Autodesk Inventor part; units mm, degrees
ref_plane "YZ Plane" through (0, 0, 0) normal (1, 0, 0) x (0, 1, 0)
ref_plane "XZ Plane" through (0, 0, 0) normal (0, 1, 0) x (-1, 0, 0)
ref_plane "XY Plane" through (0, 0, 0) normal (0, 0, 1) x (1, 0, 0)
sketch "Náčrt1" plane through (0, 0, 0) normal (0, 1, 0) x (-1, 0, 0)
  line L0 (0, 0) -> (-75, 0)
  line L1 (-75, 0) -> (-75, -60)
  line L2 (-75, -60) -> (0, -60)
  line L3 (0, -60) -> (0, 0)
  line L4 (2, 2) -> (-77, 2)
  line L5 (-77, 2) -> (-77, -62)
  line L6 (-77, -62) -> (2, -62)
  line L7 (2, -62) -> (2, 2)
  dimension "d0" = 60
  dimension "d1" = 75
  dimension "d2" = 2
  dimension "d3" = 2
  dimension "d4" = 2
  dimension "d5" = 2
extrude "Vysunutí1" add sketch "Náčrt1" along normal blind 2 contours L3 L2 L1 L0
extrude "Vysunutí2" add sketch "Náčrt1" along normal blind 32
sketch "Náčrt2" plane through (0, 32, 0) normal (0, 1, 0) x (1, 0, 0)
  line L0 (-2, -2) -> (4, -2)
  line L1 (4, -2) -> (4, 4)
  line L2 (4, 4) -> (-2, 4)
  line L3 (-2, 4) -> (-2, -2)
  line L4 (77, 62) -> (-2, 62)
  line L5 (-2, 62) -> (4, 62)
  line L6 (4, 62) -> (4, 56)
  line L7 (4, 56) -> (-2, 56)
  line L8 (-2, 56) -> (-2, 62)
  line L9 (77, -2) -> (77, 62)
  line L10 (77, 62) -> (71, 62)
  line L11 (71, 62) -> (71, 56)
  line L12 (71, 56) -> (77, 56)
  line L13 (77, 56) -> (77, 62)
  line L14 (77, -2) -> (71, -2)
  line L15 (71, -2) -> (71, 4)
  line L16 (71, 4) -> (77, 4)
  line L17 (77, 4) -> (77, -2)
  point P0 (0, 0)
  dimension "d10" = 6
  dimension "d11" = 6
  dimension "d12" = 6
  dimension "d13" = 6
  dimension "d14" = 6
  dimension "d15" = 6
  dimension "d16" = 6
  dimension "d17" = 6
extrude "Vysunutí3" add sketch "Náčrt2" against normal blind 10
sketch "Náčrt3" plane through (0, 32, 0) normal (0, 1, 0) x (1, 0, 0)
  circle A0 centre (1.5, 58.5) radius 1
  line L0 (77, 62) -> (-2, 62)
  line L1 (-2, 62) -> (-2, -2)
  circle A1 centre (73.5, 58.5) radius 1
  line L2 (77, -2) -> (77, 62)
  circle A2 centre (73.5, 1.5) radius 1
  line L3 (-2, -2) -> (77, -2)
  circle A3 centre (1.5, 1.5) radius 1
  point P0 (0, 0)
  dimension "d20" = 2
  dimension "d21" = 3.5
  dimension "d22" = 3.5
  dimension "d23" = 2
  dimension "d24" = 3.5
  dimension "d25" = 3.5
  dimension "d26" = 2
  dimension "d27" = 3.5
  dimension "d28" = 3.5
  dimension "d29" = 2
  dimension "d30" = 3.5
  dimension "d31" = 3.5
extrude "Vysunutí4" cut sketch "Náčrt3" against normal blind 10 contours A0 | A1 | A2 | A3
sketch "Náčrt4" plane through (77, 0, 2) normal (1, 0, 0) x (0, 0, -1)
  line L0 (2, 2) -> (2, 22)
  line L1 (6.5, 5.7) -> (15, 5.7)
  line L2 (15, 5.7) -> (15, 3)
  line L3 (15, 3) -> (6.5, 3)
  line L4 (6.5, 3) -> (6.5, 5.7)
  line L5 (0, 0) -> (64, 0)
  point P0 (2, 0)
  dimension "d36" = 3
  dimension "d37" = 4.5
  dimension "d38" = 8.5
  dimension "d39" = 2.7
extrude "Vysunutí5" cut sketch "Náčrt4" against normal blind 10
sketch "Náčrt5" plane through (75, 2, -60) normal (-1, 0, 0) x (0, 0, 1)
  line L0 (60, 0) -> (0, 0)
  line L1 (42.65, 1) -> (60, 1)
  line L2 (60, 1) -> (60, 0)
  line L3 (60, 0) -> (42.65, 0)
  line L4 (42.65, 0) -> (42.65, 1)
  line L5 (60, 0) -> (60, 20)
  point P0 (60, -2)
  point P1 (60, 0.5)
  point P2 (42.65, 0)
  dimension "d42" = 17.35
  dimension "d43" = 1
extrude "Vysunutí6" cut sketch "Náčrt5" against normal blind 1
chamfer "Zkosení1" distance 0.5 angle 45 5 edges at (75.5, 3, -13) (75.5, 3, -4.5) (75, 4.35, -4.5) (75, 4.35, -13) (75, 5.7, -8.75)
chamfer "Zkosení2" distance 0.5 angle 45 4 edges at (77, 5.7, -8.75) (77, 4.35, -4.5) (77, 3, -8.75) (77, 4.35, -13)
sketch "Náčrt6" plane through (77, 0, 2) normal (1, 0, 0) x (0, 0, -1)
  point P0 (2, 0)
fillet "Zaoblení1" radius 2 4 edges at (77, 16, 2) (77, 16, -62) (-2, 16, -62) (-2, 16, 2)
equation "\"d3\" = d2"
equation "\"d4\" = d2"
equation "\"d5\" = d2"
equation "\"d12\" = d10"
equation "\"d13\" = d10"
equation "\"d14\" = d10"
equation "\"d15\" = d10"
equation "\"d16\" = d10"
equation "\"d23\" = d20"
equation "\"d24\" = d21"
equation "\"d25\" = d21"
equation "\"d26\" = d20"
equation "\"d27\" = d21"
equation "\"d28\" = d21"
equation "\"d29\" = d20"
equation "\"d30\" = d21"
equation "\"d31\" = d21"
properties part number "BH1750-case" material "PVC potrubí"
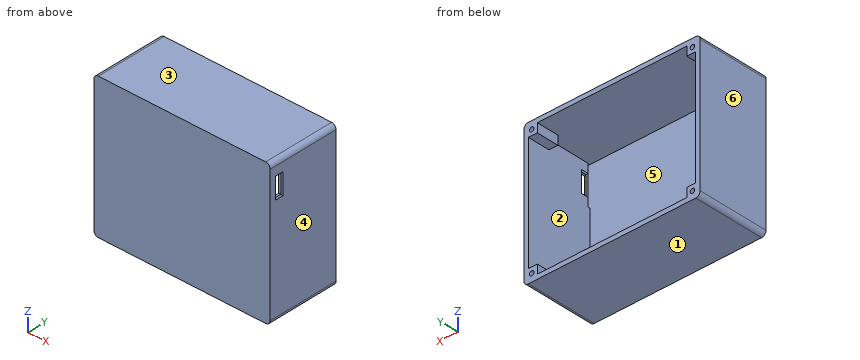
Could you check a few things on this model? Use its own coordinates, in mm. Face numbers are marked on the shaded views. A direction names the side the tool comes from. Coordinates: 2 decimals unless noted, no trailing zeros. Loops run counter-clockwise (first coordinate to the right, second up) from the corner with the lowest first, then second, coordinate; pieces in that order, holes last. Notation, with made-up numbers: (60.5, -37.5) -> (97.5, -37.5) arc R25 cw to (97.5, -21.5) -> close; hole circle Ø8 at (73, 55). An arc over 180 degrees is marked (long way). Answer in a Markdown table with one row per item.
(1) Will these pins go through, and if not, where does the flat tip stop? pin 1 Ø1.6 at (x, z) = (73.5, -58.5) entering from -Y; pin 2 Ø0.8 at (x, y) = (76, 4) entering from -Z; pin 3 Ø0.8 at (x, y) = (76, 4.5) entering from +Z.
Results found:
| item | result |
|---|---|
| pin 1 | stops at y = 0 |
| pin 2 | stops at z = -61.91 |
| pin 3 | stops at z = 1.91 |
(2) For the marked faces 1 and 2, which set-ups out of +Z, -Z, +X, -X, +Y, -Y let a thin tool reach every point of the face, with its end or its side?
Results found:
| item | result |
|---|---|
| face 1 | -Z, +X, -X, +Y, -Y |
| face 2 | none |
(3) If I drill on probe 1 along X at (y, z) = (27.5, -1.5); probe 2 along Z at (x, y) = (73.5, 24.75); probe 3 along Z at (x, y) = (47, 12), over which ranges is the centre line in solid material (lowest first)?
Results found:
| item | result |
|---|---|
| probe 1 | x = -2 to 0.5, 2.5 to 4, 71 to 72.5, 74.5 to 77 |
| probe 2 | z = -62 to -59.5, -57.5 to -56, -4 to -2.5, -0.5 to 2 |
| probe 3 | z = -62 to -60, 0 to 2 |
(4) Imagine slicing it at C-C (y = 17). List the corners of the cut face in (x, z) for me, plus the area to 3 significant figures.
Results found:
| item | result |
|---|---|
| outline | (-2, -60) arc R2 ccw to (0, -62) -> (75, -62) arc R2 ccw to (77, -60) -> (77, 0) arc R2 ccw to (75, 2) -> (0, 2) arc R2 ccw to (-2, 0) -> close; hole (0, -60) -> (75, -60) -> (75, 0) -> (0, 0) -> close |
| area | 553 mm^2 |
(5) Thinking about a two-plate mould opening in X: for the marked faces 3, 4, 5 and 6, which applies, released by +X, released by -X, zero draft, split by the parting line, or undercut?
Results found:
| item | result |
|---|---|
| face 3 | zero draft |
| face 4 | released by +X |
| face 5 | undercut |
| face 6 | released by -X |
(6) Imagine slicing it at D-D (z = -6.5). List the corners of the cut face in (x, y) for me.
Results found:
| item | result |
|---|---|
| outline | (-2, 0) -> (77, 0) -> (77, 2.5) -> (76.5, 3) -> (76, 3) -> (76, 2) -> (0, 2) -> (0, 32) -> (-2, 32) -> close; (75, 6.2) -> (75.5, 5.7) -> (76.5, 5.7) -> (77, 6.2) -> (77, 32) -> (75, 32) -> close |
(7) Imagine slicing it at B-B (x = 73.5). List the corners of the cut face in (y, z) for me.
Results found:
| item | result |
|---|---|
| outline | (0, -62) -> (32, -62) -> (32, -59.5) -> (22, -59.5) -> (22, -60) -> (2, -60) -> (2, 0) -> (22, 0) -> (22, -0.5) -> (32, -0.5) -> (32, 2) -> (0, 2) -> close; (22, -57.5) -> (32, -57.5) -> (32, -56) -> (22, -56) -> close; (22, -4) -> (32, -4) -> (32, -2.5) -> (22, -2.5) -> close |
(8) Imagine slicing it at A-A (z = -58.5). List the corners of the cut face in (x, y) for me.
Results found:
| item | result |
|---|---|
| outline | (-2, 0) -> (77, 0) -> (77, 32) -> (74.5, 32) -> (74.5, 22) -> (75, 22) -> (75, 2) -> (0, 2) -> (0, 22) -> (0.5, 22) -> (0.5, 32) -> (-2, 32) -> close; (2.5, 22) -> (4, 22) -> (4, 32) -> (2.5, 32) -> close; (71, 22) -> (72.5, 22) -> (72.5, 32) -> (71, 32) -> close |
